from build123d import *

# Parameters (mm, degrees)
SKETCH1_W             = 10
SKETCH1_H             = 5
BOSS_EXTRUDE1_DEPTH   = 21
BOSS_EXTRUDE1_2_DEPTH = 21
BOSS_EXTRUDE2_DEPTH   = 6
SKETCH3_W             = 20.5
SKETCH3_H             = 5
BOSS_EXTRUDE3_DEPTH   = 21
CUT_EXTRUDE1_REACH    = 64.414
SKETCH4_R             = 1.65
CUT_EXTRUDE2_REACH    = 61.08
SKETCH5_R             = 2.2
SKETCH6_R             = 1.75
BOSS_EXTRUDE4_DEPTH   = 6
CUT_EXTRUDE3_REACH    = 107.857
CUT_EXTRUDE7_REACH    = 109.208
BOSS_EXTRUDE5_DEPTH   = 6
BOSS_EXTRUDE6_DEPTH   = 3
BOSS_EXTRUDE7_DEPTH   = 3
BOSS_EXTRUDE8_DEPTH   = 20.5
SKETCH16_W            = 61.423716469
SKETCH16_H            = 45.352356837
CUT_EXTRUDE8_DEPTH    = 21
CUT_EXTRUDE9_DEPTH    = 6
FILLET1_R             = 1
CUT_EXTRUDE10_DEPTH   = 2


with BuildPart() as part:
    # Sketch1 → Boss-Extrude1 (new body)
    with BuildSketch(Plane.XY):
        with Locations((-31.296703297, 19.79010989)):
            Rectangle(SKETCH1_W, SKETCH1_H)
    boss_extrude1 = extrude(amount=BOSS_EXTRUDE1_DEPTH)



with BuildPart() as body_2:
    # Sketch1 → Boss-Extrude1 2 (new body)
    with BuildSketch(Plane.XY):
        with Locations((19.703296703, 19.79010989)):
            Rectangle(SKETCH1_W, SKETCH1_H)
    boss_extrude1_2 = extrude(amount=BOSS_EXTRUDE1_2_DEPTH)


with BuildPart() as part_1:
    add(part.part)

    add(body_2.part)  # Boss-Extrude2 merges body 2
    # Sketch2 → Boss-Extrude2 (add)
    with BuildSketch(Plane.XY.offset(21)):
        Polygon((-36.296703297, 22.29010989), (24.703296703, 22.29010989), (24.703296703, 7.29010989), (12.703296703, 7.29010989), (-5.796703297, -11.20989011), (-5.796703297, -20.70989011), (-36.296703297, -20.70989011), align=None)
    extrude(amount=BOSS_EXTRUDE2_DEPTH)

    # Sketch3 → Boss-Extrude3 (add)
    with BuildSketch(Plane(origin=(0, 0, 21), x_dir=(-1, 0, 0), z_dir=(0, 0, -1))):
        with Locations((16.046703297, -18.20989011)):
            Rectangle(SKETCH3_W, SKETCH3_H)
    boss_extrude3 = extrude(amount=BOSS_EXTRUDE3_DEPTH)

    # Sketch4 → Cut-Extrude1 (cut, up to next)
    with BuildSketch(Plane(origin=(0, 22.29010989, 0), x_dir=(1, 0, 0), z_dir=(0, 1, 0)), mode=Mode.PRIVATE) as cut_extrude1_sk1:
        with Locations(Location((-29.796703297, -5.5, 0), (0, 0, 270))):
            Circle(SKETCH4_R)
    cut_extrude1_tool1 = extrude(cut_extrude1_sk1.sketch, amount=-CUT_EXTRUDE1_REACH, mode=Mode.PRIVATE) & part_1.part
    # Sketch4 → Cut-Extrude1 (cut, up to next)
    with BuildSketch(Plane(origin=(0, 22.29010989, 0), x_dir=(1, 0, 0), z_dir=(0, 1, 0)), mode=Mode.PRIVATE) as cut_extrude1_sk2:
        with Locations(Location((18.203296703, -5.5, 0), (0, 0, 270))):
            Circle(SKETCH4_R)
    cut_extrude1_tool2 = extrude(cut_extrude1_sk2.sketch, amount=-CUT_EXTRUDE1_REACH, mode=Mode.PRIVATE) & part_1.part
    # Sketch4 → Cut-Extrude1 (cut, up to next)
    with BuildSketch(Plane(origin=(0, 22.29010989, 0), x_dir=(1, 0, 0), z_dir=(0, 1, 0)), mode=Mode.PRIVATE) as cut_extrude1_sk3:
        with Locations(Location((18.203296703, -15.5, 0), (0, 0, 270))):
            Circle(SKETCH4_R)
    cut_extrude1_tool3 = extrude(cut_extrude1_sk3.sketch, amount=-CUT_EXTRUDE1_REACH, mode=Mode.PRIVATE) & part_1.part
    # Sketch4 → Cut-Extrude1 (cut, up to next)
    with BuildSketch(Plane(origin=(0, 22.29010989, 0), x_dir=(1, 0, 0), z_dir=(0, 1, 0)), mode=Mode.PRIVATE) as cut_extrude1_sk4:
        with Locations(Location((-29.796703297, -15.5, 0), (0, 0, 270))):
            Circle(SKETCH4_R)
    cut_extrude1_tool4 = extrude(cut_extrude1_sk4.sketch, amount=-CUT_EXTRUDE1_REACH, mode=Mode.PRIVATE) & part_1.part
    cut_extrude1_1 = cut_extrude1_tool1.solids().sort_by_distance((-29.796703, 22.29011, 5.5))[0]
    add(cut_extrude1_1, mode=Mode.SUBTRACT)
    cut_extrude1_2 = cut_extrude1_tool2.solids().sort_by_distance((18.203297, 22.29011, 5.5))[0]
    add(cut_extrude1_2, mode=Mode.SUBTRACT)
    cut_extrude1_3 = cut_extrude1_tool3.solids().sort_by_distance((18.203297, 22.29011, 15.5))[0]
    add(cut_extrude1_3, mode=Mode.SUBTRACT)
    cut_extrude1_4 = cut_extrude1_tool4.solids().sort_by_distance((-29.796703, 22.29011, 15.5))[0]
    add(cut_extrude1_4, mode=Mode.SUBTRACT)
    cut_extrude1 = cut_extrude1_1 + cut_extrude1_2 + cut_extrude1_3 + cut_extrude1_4  # Cut-Extrude1 as one shape, for the pattern or mirror that repeats it

    # Sketch5 → Cut-Extrude2 (cut, up to next)
    with BuildSketch(Plane(origin=(0, -15.70989011, 0), x_dir=(1, 0, 0), z_dir=(0, 1, 0)), mode=Mode.PRIVATE) as cut_extrude2_sk1:
        with Locations(Location((-16.046703297, -10.5, 0), (0, 0, 270))):
            Circle(SKETCH5_R)
    cut_extrude2_tool1 = extrude(cut_extrude2_sk1.sketch, amount=-CUT_EXTRUDE2_REACH, mode=Mode.PRIVATE) & part_1.part
    cut_extrude2 = cut_extrude2_tool1.solids().sort_by_distance((-16.046703, -15.70989, 10.5))[0]
    add(cut_extrude2, mode=Mode.SUBTRACT)

    # Sketch6 → Boss-Extrude4 (add)
    with BuildSketch(Plane.XY.offset(27)):
        with BuildLine():
            Line((-79.859138265, -39.735236509), (-51.503727763, -19.880564327))
            add(Edge.make_bspline(
                [(-51.503727763, -19.880564327), (-43.777944292, -18.491061957), (-36.296703297, -20.70989011)],
                knots=[0, 0, 0, 1, 1, 1], degree=2))
            Line((-36.296703297, -20.70989011), (-36.296703297, 22.29010989))
            add(Edge.make_bspline(
                [(-57.962836939, 19.661219133), (-46.447122218, 13.814864777), (-36.296703297, 22.29010989)],
                knots=[0, 0, 0, 1, 1, 1], degree=2))
            add(Edge.make_bspline(
                [(-95.842115451, -15.524174544), (-74.663700283, -0.348148579), (-57.962836939, 19.661219133)],
                knots=[0, 0, 0, 1, 1, 1], degree=2))
            add(Edge.make_bspline(
                [(-95.842115451, -15.524174544), (-85.086697095, -25.754599345), (-79.859138265, -39.735236509)],
                knots=[0, 0, 0, 1, 1, 1], degree=2))
        make_face()
        with Locations((-40.590214383, -0.641481396)):
            Circle(SKETCH6_R, mode=Mode.SUBTRACT)
        with Locations((-85.645276872, -19.981629898)):
            Circle(SKETCH6_R, mode=Mode.SUBTRACT)
        with Locations((-79.909512508, -28.173150341)):
            Circle(SKETCH6_R, mode=Mode.SUBTRACT)
        with Locations((-46.325978746, 7.550039047)):
            Circle(SKETCH6_R, mode=Mode.SUBTRACT)
        Polygon((-85.932915117, -13.468776127), (-52.347681301, 10.047857763), (-40.302576138, -7.154335167), (-73.887809953, -30.670969058), align=None, mode=Mode.SUBTRACT)
    extrude(amount=-BOSS_EXTRUDE4_DEPTH)

    # Sketch7 → Cut-Extrude3 (cut, up to next)
    with BuildSketch(Plane(origin=(0, 0, 21), x_dir=(-1, 0, 0), z_dir=(0, 0, -1)), mode=Mode.PRIVATE) as cut_extrude3_sk1:
        with BuildLine():
            Line((36.296703297, -20.70989011), (26.296703297, -20.70989011))
            add(Edge.make_bspline(
                [(26.296703297, -20.70989011), (39.15974316, -13.056772406), (51.503727763, -19.880564327)],
                knots=[0, 0, 0, 1, 1, 1], degree=2))
            add(Edge.make_bspline(
                [(51.503727763, -19.880564327), (43.777944292, -18.491061957), (36.296703297, -20.70989011)],
                knots=[0, 0, 0, 1, 1, 1], degree=2))
        make_face()
    cut_extrude3_tool1 = extrude(cut_extrude3_sk1.sketch, amount=-CUT_EXTRUDE3_REACH, mode=Mode.PRIVATE) & part_1.part
    add(cut_extrude3_tool1.solids().sort_by_distance((-38.072503, -18.786508, 21))[0], mode=Mode.SUBTRACT)

    # Sketch10 → Cut-Extrude7 (cut, up to next)
    with BuildSketch(Plane.XY.offset(27), mode=Mode.PRIVATE) as cut_extrude7_sk1:
        with BuildLine():
            Line((5.266834936, 14.29010989), (-27.788194587, 14.29010989))
            add(Edge.make_bspline(
                [(-27.788194587, 14.29010989), (-23.431396766, 3.132914333), (-25.823714091, -8.70989011)],
                knots=[0, 0, 0, 1, 1, 1], degree=2))
            Line((-25.823714091, -8.70989011), (-13.796703297, -8.70989011))
            add(Edge.make_bspline(
                [(5.266834936, 14.29010989), (-9.842167425, 7.185288479), (-13.796703297, -8.70989011)],
                knots=[0, 0, 0, 1, 1, 1], degree=2))
        make_face()
    cut_extrude7_tool1 = extrude(cut_extrude7_sk1.sketch, amount=-CUT_EXTRUDE7_REACH, mode=Mode.PRIVATE) & part_1.part
    add(cut_extrude7_tool1.solids().sort_by_distance((-15.764918, 4.836925, 27))[0], mode=Mode.SUBTRACT)

    # Sketch11 → Boss-Extrude5 (add)
    with BuildSketch(Plane.XY.offset(27)):
        with BuildLine():
            Line((15.119169314, 7.29010989), (12.703296703, 7.29010989))
            Line((12.703296703, 7.29010989), (-5.796703297, -11.20989011))
            Line((-5.796703297, -11.20989011), (-5.796703297, -20.70989011))
            add(Edge.make_bspline(
                [(-5.796703297, -20.70989011), (-0.06692684, -3.022661062), (15.119169314, 7.29010989)],
                knots=[0, 0, 0, 1, 1, 1], degree=2))
        make_face()
    extrude(amount=-BOSS_EXTRUDE5_DEPTH)

    # Sketch12 → Boss-Extrude6 (add)
    with BuildSketch(Plane(origin=(24.703296703, 0, 0), x_dir=(0, 0, -1), z_dir=(1, 0, 0))):
        Polygon((-21, 11.29010989), (-9, 17.29010989), (-21, 17.29010989), align=None)
    boss_extrude6 = extrude(amount=-BOSS_EXTRUDE6_DEPTH)

    # Sketch13 → Boss-Extrude7 (add)
    with BuildSketch(Plane.ZY.offset(36.296703297)):
        Polygon((21, 11.29010989), (21, 17.29010989), (9, 17.29010989), align=None)
    boss_extrude7 = extrude(amount=-BOSS_EXTRUDE7_DEPTH)

    # Sketch14 → Boss-Extrude8 (add)
    with BuildSketch(Plane(origin=(-5.796703297, 0, 0), x_dir=(0, 0, -1), z_dir=(1, 0, 0))):
        Polygon((-17.7, -15.70989011), (-21, -12.40989011), (-21, -15.70989011), align=None)
    boss_extrude8 = extrude(amount=-BOSS_EXTRUDE8_DEPTH)

    # Mirror1: Boss-Extrude1, Boss-Extrude1 2, Boss-Extrude3, Cut-Extrude1, Cut-Extrude2, Boss-Extrude6, Boss-Extrude7, Boss-Extrude8 across plane
    add(boss_extrude1.mirror(Plane(origin=(0, 0, 24), x_dir=(1, 0, 0), z_dir=(0, 0, -1))))
    add(boss_extrude1_2.mirror(Plane(origin=(0, 0, 24), x_dir=(1, 0, 0), z_dir=(0, 0, -1))))
    add(boss_extrude3.mirror(Plane(origin=(0, 0, 24), x_dir=(1, 0, 0), z_dir=(0, 0, -1))))
    add(cut_extrude1.mirror(Plane(origin=(0, 0, 24), x_dir=(1, 0, 0), z_dir=(0, 0, -1))), mode=Mode.SUBTRACT)
    add(cut_extrude2.mirror(Plane(origin=(0, 0, 24), x_dir=(1, 0, 0), z_dir=(0, 0, -1))), mode=Mode.SUBTRACT)
    add(boss_extrude6.mirror(Plane(origin=(0, 0, 24), x_dir=(1, 0, 0), z_dir=(0, 0, -1))))
    add(boss_extrude7.mirror(Plane(origin=(0, 0, 24), x_dir=(1, 0, 0), z_dir=(0, 0, -1))))
    add(boss_extrude8.mirror(Plane(origin=(0, 0, 24), x_dir=(1, 0, 0), z_dir=(0, 0, -1))))

    # Sketch16 → Cut-Extrude8 (cut)
    with BuildSketch(Plane(origin=(0, 0, 0), x_dir=(-1, 0, 0), z_dir=(0, 0, -1))):
        with Locations((6.008561531, -0.386068529)):
            Rectangle(SKETCH16_W, SKETCH16_H)
    extrude(amount=-CUT_EXTRUDE8_DEPTH, mode=Mode.SUBTRACT)

    # Sketch17 → Cut-Extrude9 (cut)
    with BuildSketch(Plane(origin=(0, 0, 21), x_dir=(-1, 0, 0), z_dir=(0, 0, -1))):
        with BuildLine():
            Line((-24.703296703, 7.29010989), (-24.703296703, 11.09010989))
            add(Edge.make_bspline(
                [(5.796703297, -20.70989011), (-1.890928929, 9.845343686), (-24.703296703, 11.09010989)],
                knots=[0, 0, 0, 1, 1, 1], degree=2))
            add(Edge.make_bspline(
                [(5.796703297, -20.70989011), (0.06692684, -3.022661062), (-15.119169314, 7.29010989)],
                knots=[0, 0, 0, 1, 1, 1], degree=2))
            Line((-15.119169314, 7.29010989), (-24.703296703, 7.29010989))
        make_face()
    extrude(amount=-CUT_EXTRUDE9_DEPTH, mode=Mode.SUBTRACT)

    # Fillet1
    fillet1_edges = [part_1.edges().sort_by_distance(p)[0] for p in [
        (-79.859138265, -39.735236509, 24),
        (-95.842115451, -15.524174544, 24),
        (-57.962836939, 19.661219133, 24),
    ]]
    fillet(fillet1_edges, radius=FILLET1_R)

    # Sketch18 → Cut-Extrude10 (cut)
    with BuildSketch(Plane(origin=(0, -15.70989011, 0), x_dir=(1, 0, 0), z_dir=(0, 1, 0))):
        Polygon((-18.182899293, -41.2), (-13.910507301, -41.2), (-11.774311305, -37.5), (-13.910507301, -33.8), (-18.182899293, -33.8), (-20.319095289, -37.5), align=None)
    extrude(amount=-CUT_EXTRUDE10_DEPTH, mode=Mode.SUBTRACT)


solid = part_1.part
Work out the finished part from the listing and answer in its coordinate system (mm). A direction names the side the tool comes from. Coordinates: 2 decimals unless noted, no trailing zeros. Loops run counter-clockwise (first coordinate to the right, second up) from the corner with the lowest first, then second, coordinate; pieces in that order, holes last. Notation, with made-up numbers: (69, 1.5) -> (77, 1.5) arc R34 ccw to (77, 40.5) -> close; hole circle Ø4 at (-20.5, -38.5). An arc over 180 degrees is marked (long way). Write each question's results on one line, items separated by ' | '. Start each with the question number.
1) Flat-ended cylindrical pins translate along their axes: P1, Ø2.5, axis at y = -17.5, z = 41.5, coming from the -X side; P2, Ø8, axis at x = -74.5, y = -4, coming from the +Z side; P3, Ø12, axis at y = 14, z = 45, coming from the -X side. Find the tip coordinate at first contact, or state that the pin passes through.
2) The mould has two halves that part along X. Classify faces 4 (the flat face through (-16, -18, 48)), 5 (the flat face through (-36.297, 18, 35)), 6 (the flat face through (-5.797, -18, 37)), 7 (the flat face through (-69.38, -1.88, 24.04)): pulls with the +X half, pulls with the -X half, needs draft (parallel to the pull), parting line crosses it, or undercut.
3) Consider line 1 along X through (y, z) = (20, 42.5); line 2 along X through (y, z) = (20, 37.5); line 3 along X through (y, z) = (-19.2, 37.5). Determine where each line is inside the solid, lowest interval first.
4) Find section B-B on z = 32.5. Determine the outline of the cut face in (x, y), then the cut area to 3 significant figures.
5) Find section C-C on z = 24.25. Count the separate pieces of the cut face and the enclosed holes in it, then the cut area to 3 significant figures.
6) Find section A-A on z = 46. Determine the outline of the cut face in (x, y), then the cut area to 4 significant figures.
7) For faces 1 (the flat face through (-26.297, 20, 38)), 2 (the flat face through (-19.236, -16.696, 35.624)), 3 (the flat face through (-56.86, -18.75, 24.04)), determine the directions among +Z, -Z, +X, -X, +Y, -Y from which every point of the face is accessible in a straight line to the end or side of a thin tool.
Response values:
1) P1: stops at x = -26.3 | P2: stops at z = 27 | P3: stops at x = -36.3
2) face 4: needs draft | face 5: pulls with the -X half | face 6: pulls with the +X half | face 7: undercut
3) line 1: x = -36.3 to -31.45, -28.15 to -26.3, 14.7 to 16.55, 19.85 to 24.7 | line 2: x = -36.3 to -26.3, 14.7 to 24.7 | line 3: x = -26.3 to -18.25, -13.85 to -5.8
4) outline: (-36.3, 14.04) -> (-33.3, 14.04) -> (-33.3, 17.29) -> (-31.45, 17.29) -> (-31.45, 22.29) -> (-36.3, 22.29) -> close; (-28.15, 17.29) -> (-26.3, 17.29) -> (-26.3, 22.29) -> (-28.15, 22.29) -> close; (-26.3, -20.71) -> (-5.8, -20.71) -> (-5.8, -15.71) -> (-26.3, -15.71) -> close; (14.7, 17.29) -> (16.55, 17.29) -> (16.55, 22.29) -> (14.7, 22.29) -> close; (19.85, 17.29) -> (21.7, 17.29) -> (21.7, 14.04) -> (24.7, 14.04) -> (24.7, 22.29) -> (19.85, 22.29) -> close | area: 189 mm^2
5) separate pieces: 1 | enclosed holes: 6 | area: 2,510 mm^2
6) outline: (-36.3, 17.29) -> (-26.3, 17.29) -> (-26.3, 22.29) -> (-36.3, 22.29) -> close; (-26.3, -20.71) -> (-5.8, -20.71) -> (-5.8, -15.71) -> (-26.3, -15.71) -> close; (14.7, 17.29) -> (24.7, 17.29) -> (24.7, 22.29) -> (14.7, 22.29) -> close | area: 202.5 mm^2
7) face 1: +Z, +Y | face 2: +Y | face 3: +Z, -Z
